Read the model definition and answer for the solid it produces. Units are mm, in the model's axes. A direction names the side the tool comes from. Give positions to 0.01 mm unless a question says otherwise; leave off trailing zeros. Order: outer loops, then holes, each group sorted by start corner. A loop starts at its lowest first (then second) coordinate and runs counter-clockwise, first axis right, second up. Notation, with made-up numbers: (14.5, 75.25) - (22.5, 75.25) arc R4 cw to (22.5, 79.25) - close; hole circle Ø3 at (70, 80). An arc over 180 degrees is marked (long way). Write each question's results on one line, items separated by ' | '.
from build123d import *

# Parameters (mm, degrees)
SKETCH1_W               = 100
SKETCH1_H               = 180.7762
BASE_FLANGE1_DEPTH      = 2.032
SKETCHED_BEND1_DEPTH    = 100
SKETCHED_BEND1_2_DEPTH  = 100
SKETCHED_BEND2_DEPTH    = 100
SKETCHED_BEND2_2_DEPTH  = 100
CUT_EXTRUDE1_DEPTH      = 196.207207632
CUT_EXTRUDE1_DEPTH_BACK = 196.207207632
SKETCH1_4_R             = 1.13
F_4_40_TAPPED_HOLE1_D   = 2.2606
SKETCH11_R              = 2.5
CUT_EXTRUDE2_DEPTH      = 2.032
F_1_4_20_TAPPED_HOLE3_D = 5.1054


# Read off the part's stored shape, not the designer's step: Sketched Bend1, Sketched Bend2
# Sheet-metal steps are written as plain solids
with BuildPart() as part:
    # Sketch1 → Base-Flange1 (new body)
    with BuildSketch(Plane.XY):
        with Locations((50, -90.3881)):
            Rectangle(SKETCH1_W, SKETCH1_H)
    extrude(amount=-BASE_FLANGE1_DEPTH)

    # Sketched Bend1 outline → Sketched Bend1 (cut)
    with BuildSketch(Plane.YZ):
        with BuildLine():
            Line((-125.297528233, -0.945834787), (-126.24336302, 0))
            Line((-126.24336302, 0), (-180.7762, 0))
            Line((-180.7762, 0), (-180.7762, -2.032))
            Line((-180.7762, -2.032), (-122.675293446, -2.032))
            ThreePointArc((-122.675293446, -2.032), (-124.094436686, -1.749714858), (-125.297528233, -0.945834787))
        make_face()
    extrude(amount=SKETCHED_BEND1_DEPTH, mode=Mode.SUBTRACT)

    # Sketched Bend1 2 outline → Sketched Bend1 2 (add)
    with BuildSketch(Plane.YZ):
        with BuildLine():
            Line((-163.561829245, 40.192148183), (-164.998670225, 38.755307204))
            Line((-164.998670225, 38.755307204), (-126.24336302, 0))
            Line((-126.24336302, 0), (-122.675293446, 0))
            ThreePointArc((-122.675293446, 0), (-123.316823952, 0.127608352), (-123.860687254, 0.491006192))
            Line((-123.860687254, 0.491006192), (-163.561829245, 40.192148183))
        make_face()
    extrude(amount=SKETCHED_BEND1_2_DEPTH)

    # Sketched Bend2 outline → Sketched Bend2 (cut)
    with BuildSketch(Plane.YZ):
        with BuildLine():
            Line((-164.998670225, 38.755307204), (-149.212692342, 22.969329321))
            ThreePointArc((-149.212692342, 22.969329321), (-147.197284992, 23.051802202), (-145.43684371, 22.067162648))
            Line((-145.43684371, 22.067162648), (-163.561829245, 40.192148183))
            Line((-163.561829245, 40.192148183), (-164.998670225, 38.755307204))
        make_face()
    extrude(amount=SKETCHED_BEND2_DEPTH, mode=Mode.SUBTRACT)

    # Sketched Bend2 2 outline → Sketched Bend2 2 (add)
    with BuildSketch(Plane.YZ):
        with BuildLine():
            Line((-164.604651788, 5.270142185), (-149.244472305, 20.630321668))
            ThreePointArc((-149.244472305, 20.630321668), (-148.059078497, 21.12132786), (-146.873684689, 20.630321668))
            Line((-146.873684689, 20.630321668), (-149.212692342, 22.969329321))
            ThreePointArc((-149.212692342, 22.969329321), (-150.000143771, 22.604753197), (-150.681313284, 22.067162648))
            Line((-150.681313284, 22.067162648), (-166.041492767, 6.706983165))
            Line((-166.041492767, 6.706983165), (-164.604651788, 5.270142185))
        make_face()
    extrude(amount=SKETCHED_BEND2_2_DEPTH)

    # Sketch1<4> → Cut-Extrude1 (cut, two sides: drawn at the far end of the back side and taken through both)
    with BuildSketch(Plane.XY.offset(-CUT_EXTRUDE1_DEPTH_BACK)):
        with Locations((11.9, -7.7868)):
            Circle(SKETCH1_4_R)
        with Locations((88.1, -7.7868)):
            Circle(SKETCH1_4_R)
        with Locations((88.1, -96.6868)):
            Circle(SKETCH1_4_R)
        with Locations((11.9, -96.6868)):
            Circle(SKETCH1_4_R)
    extrude(amount=CUT_EXTRUDE1_DEPTH + CUT_EXTRUDE1_DEPTH_BACK, mode=Mode.SUBTRACT)

    # #4-40 Tapped Hole1 (through all)
    with Locations(Plane(origin=(88.1, -96.6868, 0), x_dir=(1, 0, 0), z_dir=(0, 0, 1))):
        with Locations((0, 0), (-76.2, 0), (-76.2, 88.9), (0, 88.9)):
            Hole(F_4_40_TAPPED_HOLE1_D / 2)

    # Sketch11 → Cut-Extrude2 (cut)
    with BuildSketch(Plane(origin=(0, -86.374237966, 86.374237966), x_dir=(-1, 0, 0), z_dir=(0, -0.7071067811865487, 0.7071067811865465))):
        with Locations(Location((-10, 99.966512217, 0), (0, 0, 90))):
            Circle(SKETCH11_R)
        with Locations(Location((-50, 99.966512217, 0), (0, 0, 90))):
            Circle(SKETCH11_R)
        with Locations(Location((-90, 99.966512217, 0), (0, 0, 90))):
            Circle(SKETCH11_R)
    extrude(amount=-CUT_EXTRUDE2_DEPTH, mode=Mode.SUBTRACT)

    # 1/4-20 Tapped Hole3 (through all)
    with Locations(Plane(origin=(0, -86.374237966, 86.374237966), x_dir=(-1, 0, 0), z_dir=(0, -0.7071067811865487, 0.7071067811865465))):
        with Locations((-90, 99.966512217), (-50, 99.966512217), (-10, 99.966512217)):
            Hole(F_1_4_20_TAPPED_HOLE3_D / 2)


solid = part.part
(1) The mould has two halves that part along X. Classify faces 3 (the face through (51.18, -154.73, 16.56)), 4 (the face through (100, -90, -1)), 5 (the face through (49.3, -158.739, 11.136)): pulls with the +X half, pulls with the -X half, needs draft (parallel to the pull), parting line crosses it, or undercut.
Conclusion:
face 3: undercut | face 4: pulls with the +X half | face 5: needs draft
(2) Each of these flat-tipped pins is pushed along its axis until it touches: pin 1 (3.5 mm diameter, centred on x = 11.9, y = -96.69, fed in from +Z); pin 2 (1.8 mm diameter, centred on x = 88.1, y = -7.79, fed in from +Z); pin 3 (10 mm diameter, centred on x = 61, z = 13, fed in from -Y); pin 4 (8 mm diameter, centred on x = 84.5, z = 17.5, fed in from +Y). Where does it stop, or does it pass through?
Conclusion:
pin 1: z = 0 | pin 2: through | pin 3: y = -164.75 | pin 4: y = -136.87
(3) Consider probe 1 along Y at (x, z) = (11.9, -0.75); probe 2 along Z at (x, y) = (5.5, -121); probe 3 along Y at (x, z) = (83.5, 16.5). Determine where each line is inside the solid, lowest interval first. Write a range as [from, to].
Conclusion:
probe 1: [-125.49, -97.82], [-95.56, -8.92], [-6.66, 0] | probe 2: [-2.03, 0] | probe 3: [-156.25, -153.37], [-142.74, -139.87]
(4) For faces 1 (the face through (49, -60, 0)), 2 (the face through (0, -90, -1)), determine the directions among +Z, -Z, +X, -X, +Y, -Y from which every point of the face is accessible in a straight line to the end or side of a thin tool.
Conclusion:
face 1: +Z, +X, -X, +Y | face 2: +Z, -Z, -X, +Y, -Y
(5) Section B-B (y = -11) is taken. Give the vertices of the cut face in (x, z), plus the area to 3 significant figures.
Conclusion:
outline: (0, -2.03) - (100, -2.03) - (100, 0) - (0, 0) - close | area: 203 mm^2
(6) Section A-A (x = 77) is taken. Give the vertices of the cut face in (y, z).
Conclusion:
outline: (-166.04, 6.71) - (-164.6, 5.27) - (-149.24, 20.63) arc R1.68 cw to (-146.87, 20.63) - (-125.3, -0.95) arc R3.71 ccw to (-122.68, -2.03) - (0, -2.03) - (0, 0) - (-122.68, 0) arc R1.68 cw to (-123.86, 0.49) - (-145.44, 22.07) arc R3.71 ccw to (-150.68, 22.07) - close
(7) Section C-C (y = -134.5) is taken. Give the vertices of the cut face in (x, z), plus the area to 3 significant figures.
Conclusion:
outline: (0, 8.26) - (100, 8.26) - (100, 11.13) - (0, 11.13) - close | area: 287 mm^2
